```python
from build123d import *

# Parameters (mm, degrees)
SKETCH1_R           = 15.9
BOSS_EXTRUDE1_DEPTH = 110.3
SKETCH4_R           = 20.7
BOSS_EXTRUDE4_DEPTH = 2.5
SKETCH2_W           = 2.2
SKETCH2_H           = 12.2
SKETCH2_H_2         = 2.2
SKETCH2_W_2         = 12.2
BOSS_EXTRUDE2_DEPTH = 56.375
SKETCH3_R           = 15.9
BOSS_EXTRUDE3_DEPTH = 2.5
SKETCH5_W           = 15
SKETCH5_H           = 1.651179813


with BuildPart() as part:
    # Sketch1 → Boss-Extrude1 (new body)
    with BuildSketch(Plane.XY):
        Circle(SKETCH1_R)
    extrude(amount=BOSS_EXTRUDE1_DEPTH)

    # Sketch4 → Boss-Extrude4 (add)
    with BuildSketch(Plane(origin=(0, 0, 0), x_dir=(-1, 0, 0), z_dir=(0, 0, -1))):
        Circle(SKETCH4_R)
    extrude(amount=BOSS_EXTRUDE4_DEPTH)

    # Sketch2 → Boss-Extrude2 (add)
    with BuildSketch(Plane(origin=(0, 0, -2.5), x_dir=(-1, 0, 0), z_dir=(0, 0, -1))):
        with Locations((0, 7.2)):
            Rectangle(SKETCH2_W, SKETCH2_H)
        Rectangle(SKETCH2_W, SKETCH2_H_2)
        with Locations((0, -7.2)):
            Rectangle(SKETCH2_W, SKETCH2_H)
        with Locations((7.2, 0)):
            Rectangle(SKETCH2_W_2, SKETCH2_H_2)
        with Locations((-7.2, 0)):
            Rectangle(SKETCH2_W_2, SKETCH2_H_2)
    extrude(amount=BOSS_EXTRUDE2_DEPTH)

    # Sketch3 → Boss-Extrude3 (add)
    with BuildSketch(Plane(origin=(0, 0, -58.875), x_dir=(-1, 0, 0), z_dir=(0, 0, -1))):
        Circle(SKETCH3_R)
    extrude(amount=BOSS_EXTRUDE3_DEPTH)

    # Sketch5 → Cut-Revolve4 (revolve, cut)
    with BuildSketch(Plane(origin=(0, 0, 0), x_dir=(0, 0, -1), z_dir=(1, 0, 0))):
        with Locations((51.375, 14.125589907)):
            Rectangle(SKETCH5_W, SKETCH5_H)
        Polygon((58.875, 13.3), (58.875, 5.3), (43.875, 13.3), align=None)
    revolve(axis=Axis((0, 0, 121.7025), (0, 0, -1)), mode=Mode.SUBTRACT)


solid = part.part
```
Check sheet for the modelled part. Datum: model origin and axes. Units: mm. A direction names the side the tool comes from. Give positions to 0.01 mm unless a question says otherwise; leave off trailing zeros. Loops run counter-clockwise (first coordinate to the right, second up) from the corner with the lowest first, then second, coordinate; pieces in that order, holes last. Notation, with made-up numbers: M 44.25,47 L 86.25,47 A22 cw 86.25,66 Z; hole C 32,-10 d2. An arc over 180 degrees is marked long. Answer as CSV lines item,"result".
Item 1: Draft check along Z on faces 5 (the face through (0, 0, -61.375)), 6 (the face through (-6, -15, 0)), 7 (the face through (-4, -4, -2.5)). Enter one of: pulls with the +Z half, pulls with the -Z half, needs draft (parallel to the pull), parting line crosses it, or undercut.
Reply:
face 5,"pulls with the -Z half"
face 6,"pulls with the +Z half"
face 7,"undercut"
Item 2: Set-up check for faces 1 (the face through (-7, -1.1, -30)), 2 (the face through (7, -1.1, -30)), 3 (the face through (3.45, -15.52, -60.11)), 4 (the face through (-1.1, 7, -30)): record each of +Z, -Z, +X, -X, +Y, -Y from which the full face is reachable in a straight line by a thin tool's end or side.
Reply:
face 1,"-X, -Y"
face 2,"+X, -Y"
face 3,"-Z"
face 4,"-X, +Y"
Item 3: Sectioned sample at A-A, the plane z = -25. Enter the section's corners in (x, y).
Reply:
outline,"M -13.3,-1.1 L -1.1,-1.1 L -1.1,-13.3 L 1.1,-13.3 L 1.1,-1.1 L 13.3,-1.1 L 13.3,1.1 L 1.1,1.1 L 1.1,13.3 L -1.1,13.3 L -1.1,1.1 L -13.3,1.1 Z"
Item 4: Sectioned sample at B-B, the plane z = 86. Enter the section's corners in (x, y).
Reply:
outline,"C 0,0 d31.8"
Item 5: Scan lines: L1, parallel to Z at x = 15, y = 1 (3 decimals); L2, parallel to X at y = 0.5, z = 2.5; L3, parallel to Y at x = -10, z = -6. Record each from-to range of solid material in increasing order.
Reply:
L1,"-61.375 to -58.875, -2.5 to 110.3"
L2,"-15.89 to 15.89"
L3,"-1.1 to 1.1"
Item 6: Depth check by flat-ended pin: pin 1 Ø0.7 at (y, z) = (0.5, -33) entering from -X; pin 2 Ø3.5 at (x, z) = (-5, -29.5) entering from -Y; pin 3 Ø6 at (y, z) = (-7, -38) entering from +X. Enter the tip coordinate at first touch or a pass-through.
Reply:
pin 1,"x = -13.3"
pin 2,"y = -1.1"
pin 3,"x = 1.1"
